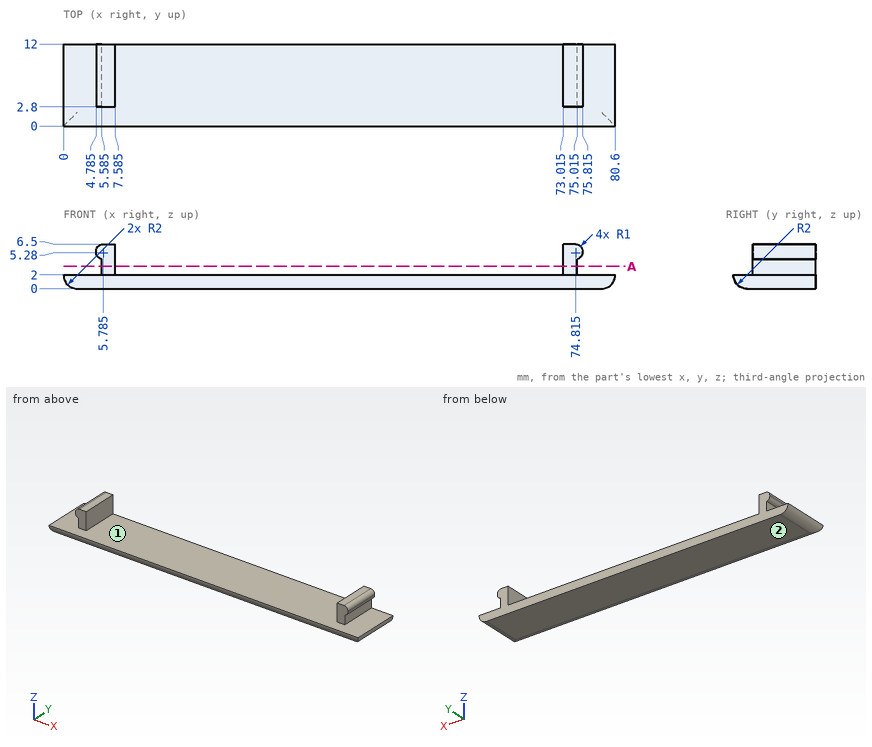
Source: three-view drawing plus pictorial views. Frame: mm from the lowest corner of the part. Round coordinates to 2 decimals unless told otherwise and drop trailing zeros. Loops run counter-clockwise (first coordinate to the right, second up) from the corner with the lowest first, then second, coordinate; pieces in that order, holes last. Notation, with made-up numbers: (44.25, 10) - (91.25, 10) arc R28 cw to (91.25, 37) - close; hole circle Ø10 at (82, -29.5). An arc over 180 degrees is marked (long way). Write item = value, one per line. Start each with the question number.
Item 1: First-contact query: pin 1 Ø1.5 at (y, z) = (6, 3) entering from +X (3 decimals); pin 2 Ø2 at (y, z) = (9.5, 5) entering from -X (3 decimals); pin 3 Ø3 at (x, z) = (74.5, 5) entering from -Y. Flat tips, straight axial feed; report the tip coordinate or a pass-through.
Item 2: Section query A-A on z = 3.25. Output: boundary loops of the cut face in (x, y) (3 decimals), plus the area to 3 significant figures.
Item 3: Mould query, pull axis X, two halves, no side actions, for the marked faces 1 and 2. Classes: released by +X, released by -X, zero draft, split by the parting line, or undercut.
Item 4: Material intervals for line 1 (X direction, y = 8, z = 3) (3 decimals); line 2 (X direction, y = 8.25, z = 5.25) (1 decimal); line 3 (Z direction, x = 30.5, y = 2.5), sorted ascending.
Results list:
q1.pin_1 = 75.015
q1.pin_2 = 4.785
q1.pin_3 = 2.8
q2.outline = (5.585, 2.8) - (7.585, 2.8) - (7.585, 12) - (5.585, 12) - close; (73.015, 2.8) - (75.015, 2.8) - (75.015, 12) - (73.015, 12) - close
q2.area = 36.8 mm²
q3.face_1 = undercut
q3.face_2 = zero draft
q4.line_1 = 5.585 to 7.585, 73.015 to 75.015
q4.line_2 = 4.8 to 7.6, 73 to 75.8
q4.line_3 = 0 to 2
